Read the model definition and answer for the solid it produces. Units are mm, in the model's axes. Give positions to 0.01 mm unless a question says otherwise; leave off trailing zeros. Order: outer loops, then holes, each group sorted by start corner. A loop starts at its lowest first (then second) coordinate and runs counter-clockwise, first axis right, second up. Notation, with made-up numbers: (-12, 19.25) - (22, 19.25) arc R32 cw to (22, 48.25) - close; hole circle Ø1 at (14.5, -29.75). An arc over 180 degrees is marked (long way). Use a Markdown table: item, result. Add a question column.
1. A cutting plane is placed at D-D on z = 11.5. Determine the outline of the cut face in (x, y) (3 decimals), and give its area (3 significant figures).
2. A cutting plane is placed at B-B on y = -1.45. Determine the outline of the cut face in (x, z) (3 decimals), and give its area (3 significant figures).
3. Flat-ended cylindrical pins translate along their axes: P1, Ø1.5, axis at x = -4, y = -2.5, coming from the +Z side; P2, Ø1, axis at y = -1.5, z = 9, coming from the +X side. Find the tip coordinate at first contact, or state that the pin passes through.
4. A cutting plane is placed at C-C on z = 7. Determine the outline of the cut face in (x, y) (3 decimals), and give its area (3 significant figures).
5. A cutting plane is placed at A-A on z = 4.25. Determine the outline of the cut face in (x, y) (3 decimals).
6. Consider L1, parallel to Z at x = -6.5, y = -0.55; L2, parallel to X at y = -2.6, z = 8.75; L3, parallel to X at y = -2.65, z = 4.5. Determine where each line is inside the solid, lowest interval first.
```python
from build123d import *

# Parameters (mm, degrees)
F1_DEPTH = 3.175
F2_R     = 5.08
F3_R     = 5.08
F4_R     = 5.08
F5_R     = 5.08


with BuildPart() as f1:
    # F0 (on Front) → F1 (new body)
    with BuildSketch(Plane.XZ):
        with BuildLine():
            Line((-12.7, 0), (-6.35, 0))
            Line((-6.35, 0), (-6.35, 3.175))
            ThreePointArc((-6.35, 3.175), (-9.525, 6.35), (-6.35, 9.525))
            Line((-6.35, 9.525), (-6.35, 12.7))
            Line((-6.35, 12.7), (-12.7, 12.7))
            Line((-12.7, 12.7), (-12.7, 0))
        make_face()
        with BuildLine():
            Line((-6.35, 0), (0, 0))
            Line((0, 0), (0, 12.7))
            Line((0, 12.7), (-6.35, 12.7))
            Line((-6.35, 12.7), (-6.35, 9.525))
            ThreePointArc((-6.35, 9.525), (-4.104936, 8.595064), (-3.175, 6.35))
            ThreePointArc((-3.175, 6.35), (-4.104936, 4.104936), (-6.35, 3.175))
            Line((-6.35, 3.175), (-6.35, 0))
        make_face()
    extrude(amount=F1_DEPTH)

    # F2
    f2_edges = [f1.edges().sort_by_distance(p)[0] for p in [
        (-12.7, -1.5875, 0),
    ]]
    fillet(f2_edges, radius=F2_R)

    # F3
    f3_edges = [f1.edges().sort_by_distance(p)[0] for p in [
        (0, -1.5875, 0),
    ]]
    fillet(f3_edges, radius=F3_R)

    # F4
    f4_edges = [f1.edges().sort_by_distance(p)[0] for p in [
        (0, -1.5875, 12.7),
    ]]
    fillet(f4_edges, radius=F4_R)

    # F5
    f5_edges = [f1.edges().sort_by_distance(p)[0] for p in [
        (-12.7, -1.5875, 12.7),
    ]]
    fillet(f5_edges, radius=F5_R)


solid = f1.part
```
Output values:
| question | item | result |
|---|---|---|
| 1 | outline | (-10.899, -3.175) - (-1.801, -3.175) - (-1.801, 0) - (-10.899, 0) - close |
| 1 | area | 28.9 mm² |
| 2 | outline | (-12.7, 5.08) arc R5.08 ccw to (-7.62, 0) - (-5.08, 0) arc R5.08 ccw to (0, 5.08) - (0, 7.62) arc R5.08 ccw to (-5.08, 12.7) - (-7.62, 12.7) arc R5.08 ccw to (-12.7, 7.62) - close; hole circle Ø6.35 at (-6.35, 6.35) |
| 2 | area | 107 mm² |
| 3 | P1 | z = 12.69 |
| 3 | P2 | x = -0.08 |
| 4 | outline | (-12.7, -3.175) - (-9.458, -3.175) - (-9.458, 0) - (-12.7, 0) - close; (-3.242, -3.175) - (0, -3.175) - (0, 0) - (-3.242, 0) - close |
| 4 | area | 20.6 mm² |
| 5 | outline | (-12.632, -3.175) - (-8.731, -3.175) - (-8.731, 0) - (-12.632, 0) - close; (-3.969, -3.175) - (-0.068, -3.175) - (-0.068, 0) - (-3.969, 0) - close |
| 6 | L1 | 0 to 3.18, 9.52 to 12.7 |
| 6 | L2 | -12.57 to -8.43, -4.27 to -0.13 |
| 6 | L3 | -12.67 to -8.93, -3.77 to -0.03 |
